Can you work these out from the model? Positions are in its coordinate system, mm. Round coordinates to 2 decimals unless told otherwise and drop trailing zeros. Order: outer loops, then holes, each group sorted by start corner. A loop starts at its lowest first (then second) coordinate and runs counter-clockwise, first axis right, second up.
Q1. If I drill on line 1 (Z direction, x = 34, y = 45); line 2 (Y direction, x = 23.5, z = 2.5); line 3 (Z direction, x = 46.5, y = 3.5), over which ranges is the centre line in solid material (lowest first)?
Q2. If we section it at B-B (y = 41): Please give me the cut outline in (x, z), plus the area to 3 significant figures.
Q3. If we section it at A-A (x = 40): Please give me the cut outline in (y, z).
Q4. If we section it at C-C (z = 5.5): Please give me the cut outline in (x, y), plus the area to 3 significant figures.
Q5. Will these pins go through, and if not, where does the flat tip stop? P1, Ø4, axis at x = 27.5, y = 48.5, coming from the +Z side; P2, Ø1, axis at x = 22, z = 4.5, coming from the +Y side; P3, Ø2, axis at x = 28, z = 2, coming from the +Y side.
from build123d import *

# Parameters (mm, degrees)
SKETCH2_W           = 54
SKETCH2_H           = 70
BOSS_EXTRUDE1_DEPTH = 5
BOSS_EXTRUDE3_DEPTH = 54
FILLET1_R           = 1


with BuildPart() as part:
    # Sketch2 → Boss-Extrude1 (new body)
    with BuildSketch(Plane.XY):
        with Locations((27, 35)):
            Rectangle(SKETCH2_W, SKETCH2_H)
    extrude(amount=-BOSS_EXTRUDE1_DEPTH)

    # Sketch6 → Boss-Extrude3 (add, through all)
    with BuildSketch(Plane(origin=(0, 0, 0), x_dir=(0, 0, -1), z_dir=(1, 0, 0))):
        Polygon((5, 0), (5, 3), (-4.451006478, 3), (-4.560038877, 4.246246021), (-7.548622971, 3.984778792), (-7.2, 0), align=None)
    extrude(amount=BOSS_EXTRUDE3_DEPTH)

    # Fillet1
    fillet1_edges = [part.edges().sort_by_distance(p)[0] for p in [
        (27, 3, 0),
        (27, 70, -5),
        (27, 3, 4.451006478),
        (27, 3.984778792, 7.548622971),
        (27, 0, 7.2),
        (27, 70, 0),
        (27, 0, -5),
    ]]
    fillet(fillet1_edges, radius=FILLET1_R)


solid = part.part
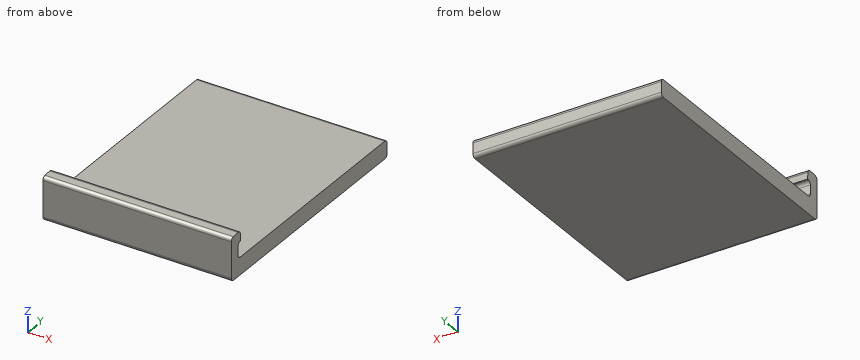
Solution:
1. line 1: z = -5 to 0
1. line 2: y = 0 to 3
1. line 3: z = -5 to 0.13, 4.4 to 7.37
2. outline: (0, -5) - (54, -5) - (54, 0) - (0, 0) - close
2. area: 270 mm2
3. outline: (0, -4) arc R1 ccw to (1, -5) - (69, -5) arc R1 ccw to (70, -4) - (70, -1) arc R1 ccw to (69, 0) - (4, 0) arc R1 cw to (3, 1) - (3, 3.53) arc R1 cw to (3.91, 4.53) - (4.25, 4.56) - (4.07, 6.55) arc R1 ccw to (2.99, 7.46) - (0.91, 7.28) arc R1 ccw to (0, 6.28) - close
4. outline: (0, 0) - (54, 0) - (54, 4.16) - (0, 4.16) - close
4. area: 225 mm2
5. P1: stops at z = 0
5. P2: stops at y = 4.25
5. P3: stops at y = 3
